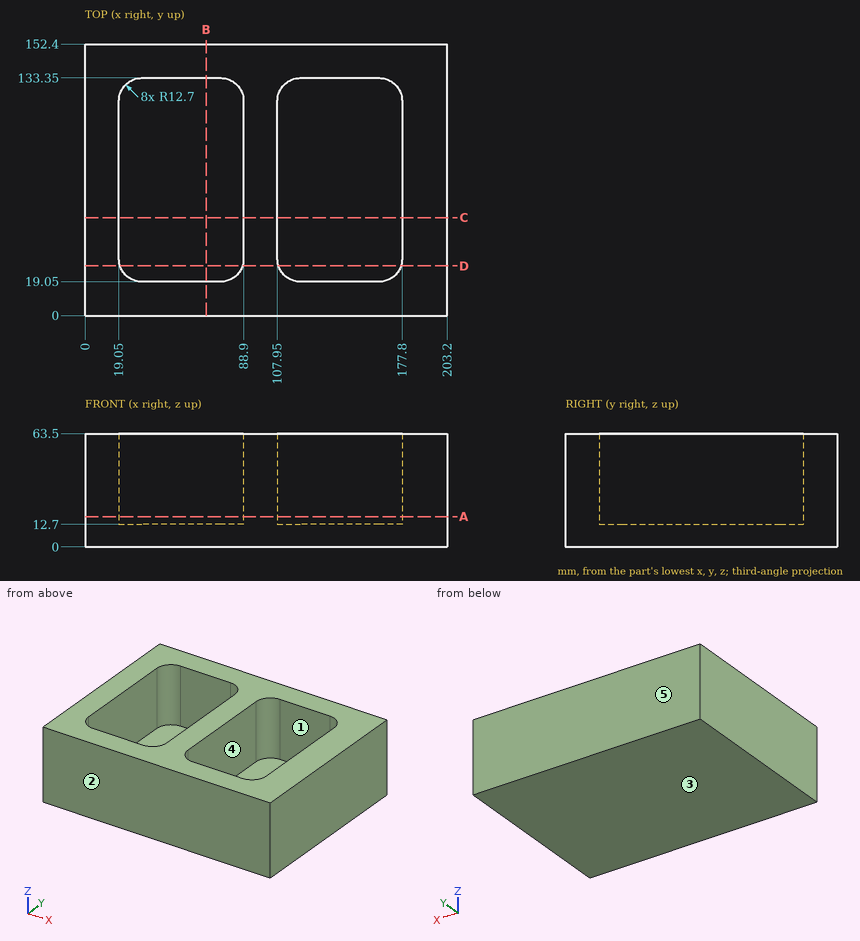
Source: three-view drawing plus pictorial views. Frame: mm from the lowest corner of the part. A direction names the side the tool comes from. Coordinates: 2 decimals unless noted, no trailing zeros. Order: outer loops, then holes, each group sorted by start corner. A loop starts at its lowest first (then second) coordinate and runs counter-clockwise, first axis right, second up.
Item 1: Cut plane C-C (y = 55). Return loops of the section in (x, z), plus the area to 3 significant figures.
Output values:
outline: (0, 0) - (203.2, 0) - (203.2, 63.5) - (177.8, 63.5) - (177.8, 12.7) - (107.95, 12.7) - (107.95, 63.5) - (88.9, 63.5) - (88.9, 12.7) - (19.05, 12.7) - (19.05, 63.5) - (0, 63.5) - close
area: 5,810 mm2
Item 2: Set-up query: the marked faces 1 and 2. Return all of +Z, -Z, +X, -X, +Y, -Y with unobstructed straight access to the full face (end or side cutting, diameter ignored); none if empty.
Output values:
face 1: +Z
face 2: +Z, -Z, +X, -X, -Y
Item 3: Cut plane D-D (y = 28). Return loops of the section in (x, z).
Output values:
outline: (0, 0) - (203.2, 0) - (203.2, 63.5) - (177.23, 63.5) - (177.23, 12.7) - (108.52, 12.7) - (108.52, 63.5) - (88.33, 63.5) - (88.33, 12.7) - (19.62, 12.7) - (19.62, 63.5) - (0, 63.5) - close
Item 4: Material intervals for line 1 (X direction, y = 75.5, z = 38); line 2 (Y direction, x = 52, z = 37); line 3 (X direction, y = 29, z = 17.5), sorted ascending.
Output values:
line 1: x = 0 to 19.05, 88.9 to 107.95, 177.8 to 203.2
line 2: y = 0 to 19.05, 133.35 to 152.4
line 3: x = 0 to 19.35, 88.6 to 108.25, 177.5 to 203.2
Item 5: Cut plane A-A (z = 17). Return loops of the section in (x, y), plus the area to 3 significant figures.
Output values:
outline: (0, 0) - (203.2, 0) - (203.2, 152.4) - (0, 152.4) - close; hole (19.05, 31.75) arc R12.7 ccw to (31.75, 19.05) - (76.2, 19.05) arc R12.7 ccw to (88.9, 31.75) - (88.9, 120.65) arc R12.7 ccw to (76.2, 133.35) - (31.75, 133.35) arc R12.7 ccw to (19.05, 120.65) - close; hole (107.95, 31.75) arc R12.7 ccw to (120.65, 19.05) - (165.1, 19.05) arc R12.7 ccw to (177.8, 31.75) - (177.8, 120.65) arc R12.7 ccw to (165.1, 133.35) - (120.65, 133.35) arc R12.7 ccw to (107.95, 120.65) - close
area: 15,300 mm2
Item 6: Pull-direction query (Y, two-part tool) for the marked faces 3, 4 and 5; classes: pulls with the +Y half, pulls with the -Y half, needs draft (parallel to the pull), parting line crosses it, or undercut.
Output values:
face 3: needs draft
face 4: undercut
face 5: pulls with the +Y half
Item 7: First-contact query: P1, Ø21, axis at x = 70, y = 100.5, coming from the +Z side. Flat tip, straight axial feed; report the tip coordinate or a pass-through.
Output values:
P1: stops at z = 12.7
Item 8: Cut plane B-B (x = 68). Return loops of the section in (y, z).
Output values:
outline: (0, 0) - (152.4, 0) - (152.4, 63.5) - (133.35, 63.5) - (133.35, 12.7) - (19.05, 12.7) - (19.05, 63.5) - (0, 63.5) - close
